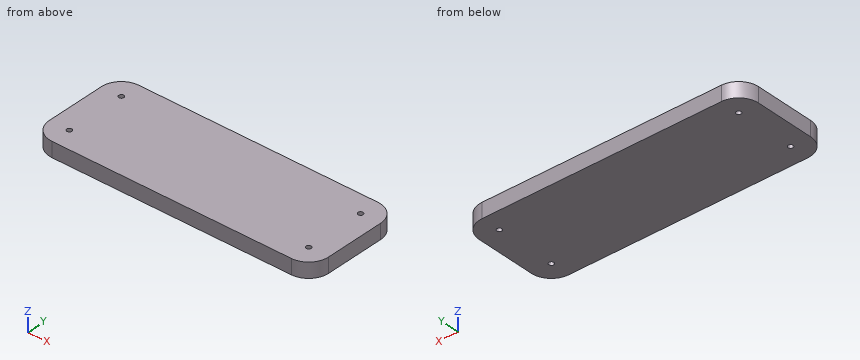
from build123d import *

# Parameters (mm, degrees)
F0_W     = 355.6
F0_H     = 127
F1_DEPTH = 19.05
F2_R     = 25.4
F3_R     = 3.175
F4_DEPTH = 19.051


with BuildPart() as f1:
    # F0 (on Top) → F1 (new body)
    with BuildSketch(Plane.XY):
        Rectangle(F0_W, F0_H)
    extrude(amount=F1_DEPTH)

    # F2
    f2_edges = [f1.edges().sort_by_distance(p)[0] for p in [
        (-177.8, 63.5, 9.525),
        (-177.8, -63.5, 9.525),
        (177.8, -63.5, 9.525),
        (177.8, 63.5, 9.525),
    ]]
    fillet(f2_edges, radius=F2_R)

    # F3 (on face) → F4 (cut, through all)
    with BuildSketch(Plane.XY.offset(19.05)):
        with Locations((-152.4, 38.1)):
            Circle(F3_R)
        with Locations((-152.4, -38.1)):
            Circle(F3_R)
        with Locations((152.4, 38.1)):
            Circle(F3_R)
        with Locations((152.4, -38.1)):
            Circle(F3_R)
    extrude(amount=-F4_DEPTH, mode=Mode.SUBTRACT)


solid = f1.part
Geometry: final body of the model. Coordinates: model frame, mm. Give positions to 0.01 mm unless a question says otherwise; leave off trailing zeros. Loops run counter-clockwise (first coordinate to the right, second up) from the corner with the lowest first, then second, coordinate; pieces in that order, holes last. Notation, with made-up numbers: M 47.5,0.5 L 102.5,0.5 A17 ccw 102.5,32.5 Z; hole C 4,48.5 d9. An arc over 180 degrees is marked long. Put each result on its own line as item: value. Start each with the question number.
1) Cut plane A-A (z = 8.5). Output: boundary loops of the cut face in (x, y) (3 decimals).
2) Contact query for flat-ended pins moving along their axis: pin 1 (2 mm diameter, centred on y = -40, z = 15, fed in from -X); pin 2 (8 mm diameter, centred on y = 42.5, z = 12.5, fed in from +X). Output: stop coordinate, or through.
3) Ray query, line 1 along Y through (x, z) = (-152.4, 14.25) (3 decimals); line 2 along X through (y, z) = (39, 4.75); line 3 along X through (y, z) = (-40.5, 6.25). Return the intervals inside material, ascending.
Verdict:
1. outline: M -177.8,-38.1 A25.4 ccw -152.4,-63.5 L 152.4,-63.5 A25.4 ccw 177.8,-38.1 L 177.8,38.1 A25.4 ccw 152.4,63.5 L -152.4,63.5 A25.4 ccw -177.8,38.1 Z; hole C -152.4,-38.1 d6.35; hole C -152.4,38.1 d6.35; hole C 152.4,-38.1 d6.35; hole C 152.4,38.1 d6.35
2. pin 1: x = -177.78
2. pin 2: x = 177.8
3. line 1: -63.5 to -41.275, -34.925 to 34.925, 41.275 to 63.5
3. line 2: -177.78 to -155.44, -149.36 to 149.36, 155.44 to 177.78
3. line 3: -177.69 to -154.48, -150.32 to 150.32, 154.48 to 177.69
